```python
from build123d import *

# Parameters (mm, degrees)
CUT_EXTRUDE3_DEPTH = 59.683963981
CUT_EXTRUDE4_DEPTH = 59.683963981
CIRPATTERN1_COUNT  = 4


with BuildPart() as part:
    # Sketch1 → Revolve1 (revolve)
    with BuildSketch(Plane(origin=(0, 0, 0), x_dir=(0, 0, -1), z_dir=(1, 0, 0)), mode=Mode.PRIVATE) as revolve1_sk:
        Polygon((-2.921, 35.449477671), (-3.937, 41.2115), (-1.778, 41.2115), (-1.2293586, 38.1), (1.2293586, 38.1), (1.778, 41.2115), (3.937, 41.2115), (2.921, 35.449477671), (2.921, 0), (-2.921, 0), align=None)
    revolve(revolve1_sk.sketch.rotate(Axis((0, 0, 2.921), (0, 0, -1)), 90), axis=Axis((0, 0, 2.921), (0, 0, -1)))

    # Sketch4 → Cut-Extrude3 (cut, through all)
    with BuildSketch(Plane(origin=(0, 0, 2.921), x_dir=(-1, 0, 0), z_dir=(0, 0, -1))):
        with BuildLine():
            Line((-3.020640994, 8.609785057), (-6.844218669, 24.749140517))
            ThreePointArc((-6.844218669, 24.749140517), (0, 33.404273107), (6.844218669, 24.749140517))
            Line((6.844218669, 24.749140517), (3.020640994, 8.609785057))
            ThreePointArc((3.020640994, 8.609785057), (0, 5.589144063), (-3.020640994, 8.609785057))
        make_face()
    cut_extrude3 = extrude(amount=CUT_EXTRUDE3_DEPTH, mode=Mode.SUBTRACT)

    # Sketch2 → Cut-Extrude4 (cut, through all)
    with BuildSketch(Plane(origin=(0, 0, 2.921), x_dir=(-1, 0, 0), z_dir=(0, 0, -1))):
        with BuildLine():
            Line((-1.397, 1.8415), (1.397, 1.8415))
            ThreePointArc((1.397, 1.8415), (3.2385, 0), (1.397, -1.8415))
            Line((1.397, -1.8415), (-1.397, -1.8415))
            ThreePointArc((-1.397, -1.8415), (-3.2385, 0), (-1.397, 1.8415))
        make_face()
    extrude(amount=CUT_EXTRUDE4_DEPTH, mode=Mode.SUBTRACT)

    # CirPattern1: Cut-Extrude3 ×4 about axis
    cirpattern1_axis = Axis((0, 0, 0), (0, 0, 1))
    for i in range(1, CIRPATTERN1_COUNT):
        add(cut_extrude3.rotate(cirpattern1_axis, i * 360 / CIRPATTERN1_COUNT), mode=Mode.SUBTRACT)


solid = part.part
```
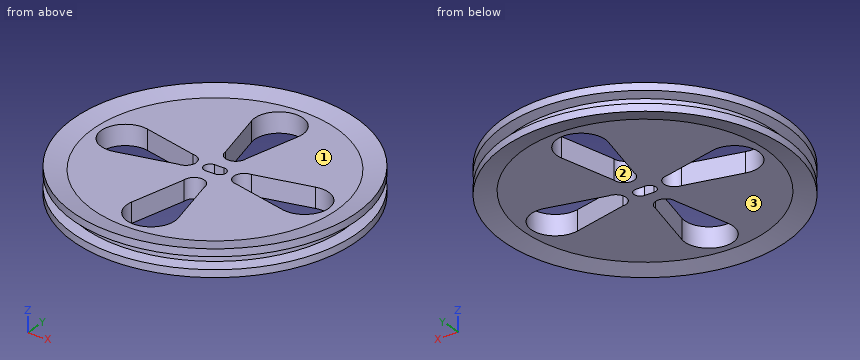
Verification items for the finished model (mm, model axes). Face numbers are marked on the shaded views. A direction names the side the tool comes from. Give positions to 0.01 mm unless a question says otherwise; leave off trailing zeros. Order: outer loops, then holes, each group sorted by start corner. A loop starts at its lowest first (then second) coordinate and runs counter-clockwise, first axis right, second up. Notation, with made-up numbers: (55, -26.5) -> (82, -26.5) arc R17 cw to (82, -18.5) -> close; hole circle Ø6 at (83, 29.5). An arc over 180 degrees is marked (long way). One line per item, written item: value.
(1) Tool access check on the marked faces 1, 2 and 3. Record the directions out of +Z, -Z, +X, -X, +Y, -Y that give a thin tool (end or side, any length) a straight path to the whole face; none if there is none.
Final values:
face 1: +Z
face 2: +Z, -Z
face 3: -Z
(2) Sectioned sample at B-B on x = 0. Record the cut outline in (y, z), then the cut area to 3 significant figures.
Final values:
outline: (-41.21, -3.94) -> (-35.45, -2.92) -> (-33.4, -2.92) -> (-33.4, 2.92) -> (-35.45, 2.92) -> (-41.21, 3.94) -> (-41.21, 1.78) -> (-38.1, 1.23) -> (-38.1, -1.23) -> (-41.21, -1.78) -> close; (-5.59, -2.92) -> (-1.84, -2.92) -> (-1.84, 2.92) -> (-5.59, 2.92) -> close; (1.84, -2.92) -> (5.59, -2.92) -> (5.59, 2.92) -> (1.84, 2.92) -> close; (33.4, -2.92) -> (35.45, -2.92) -> (41.21, -3.94) -> (41.21, -1.78) -> (38.1, -1.23) -> (38.1, 1.23) -> (41.21, 1.78) -> (41.21, 3.94) -> (35.45, 2.92) -> (33.4, 2.92) -> close
area: 128 mm^2
(3) Gauge pin test, flat ends, axial feed: pin 1 (12 mm diameter, centred on x = 16, y = 18, fed in from -Z); pin 2 (1.4 mm diameter, centred on x = 0, z = 0, fed in from +Y); pin 3 (11.5 mm diameter, centred on x = 0, y = -26.37, fed in from +Z); pin 4 (2 mm diameter, centred on y = 11, z = 1.5, fed in from +X). Record the tip position at first contact, or that the pin passes through.
Final values:
pin 1: z = -2.92
pin 2: y = 38.1
pin 3: through
pin 4: x = 39.97
(4) Sectioned sample at A-A on y = 0. Record the cut outline in (x, z), then the cut area to 3 significant figures.
Final values:
outline: (-41.21, -3.94) -> (-35.45, -2.92) -> (-33.4, -2.92) -> (-33.4, 2.92) -> (-35.45, 2.92) -> (-41.21, 3.94) -> (-41.21, 1.78) -> (-38.1, 1.23) -> (-38.1, -1.23) -> (-41.21, -1.78) -> close; (-5.59, -2.92) -> (-3.24, -2.92) -> (-3.24, 2.92) -> (-5.59, 2.92) -> close; (3.24, -2.92) -> (5.59, -2.92) -> (5.59, 2.92) -> (3.24, 2.92) -> close; (33.4, -2.92) -> (35.45, -2.92) -> (41.21, -3.94) -> (41.21, -1.78) -> (38.1, -1.23) -> (38.1, 1.23) -> (41.21, 1.78) -> (41.21, 3.94) -> (35.45, 2.92) -> (33.4, 2.92) -> close
area: 112 mm^2
(5) Scan lines: line 1 along Y through (x, z) = (0, -0.7); line 2 along X through (y, z) = (-1.5, -0.25); line 3 along Z through (x, y) = (-18, -25). Record each from-to range of solid material in increasing order. Write a range as [from, to].
Final values:
line 1: [-38.1, -33.4], [-5.59, -1.84], [1.84, 5.59], [33.4, 38.1]
line 2: [-38.07, -33.24], [-5.99, -2.47], [2.47, 5.99], [33.24, 38.07]
line 3: [-2.92, 2.92]
